```python
from build123d import *

# Parameters (mm, degrees)
SKETCH1_R           = 4
SKETCH1_R_2         = 2
BOSS_EXTRUDE1_DEPTH = 2
SKETCH3_W           = 40.799195599
SKETCH3_H           = 10.791683918
CUT_EXTRUDE1_DEPTH  = 10
SKETCH4_W           = 4.995
SKETCH4_H           = 6.450932821
BOSS_EXTRUDE2_DEPTH = 2


with BuildPart() as part:
    # Sketch1 → Boss-Extrude1 (new body)
    # profile 1 of 3: a face of its own
    with BuildSketch(Plane(origin=(0, 0, 0), x_dir=(1, 0, 0), z_dir=(0, 1, 0))):
        with BuildLine():
            ThreePointArc((26.59659241, -6.101622416), (26.022594709, -4.424555239), (26.229666852, -2.664115292))
            Line((26.229666852, -2.664115292), (10, -3.549067179))
            Line((10, -3.549067179), (-10, -3.549067179))
            Line((-10, -3.549067179), (-26.229666852, -2.664115292))
            ThreePointArc((-26.229666852, -2.664115292), (-26.057834821, -3.32225838), (-26, -4))
            ThreePointArc((-26, -4), (-26.152037529, -5.092329996), (-26.59659241, -6.101622416))
            ThreePointArc((-26.59659241, -6.101622416), (-17.96712489, -6.640913059), (-10, -10))
            Line((-10, -10), (10, -10))
            ThreePointArc((10, -10), (17.96712489, -6.640913059), (26.59659241, -6.101622416))
        make_face()
    # profile 2 of 3: a face of its own
    with BuildSketch(Plane(origin=(0, 0, 0), x_dir=(1, 0, 0), z_dir=(0, 1, 0))):
        with Locations((-30, -4)):
            Circle(SKETCH1_R)
        with Locations(Location((-30, -4, 0), (0, 0, 270))):
            Circle(SKETCH1_R_2, mode=Mode.SUBTRACT)
    # profile 3 of 3: a face of its own
    with BuildSketch(Plane(origin=(0, 0, 0), x_dir=(1, 0, 0), z_dir=(0, 1, 0))):
        with Locations((30, -4)):
            Circle(SKETCH1_R)
        with Locations(Location((30, -4, 0), (0, 0, 270))):
            Circle(SKETCH1_R_2, mode=Mode.SUBTRACT)
    extrude(amount=BOSS_EXTRUDE1_DEPTH)

    # Sketch3 → Cut-Extrude1 (cut)
    with BuildSketch(Plane(origin=(0, 2, 0), x_dir=(1, 0, 0), z_dir=(0, 1, 0))):
        with Locations((-20.3995978, -4.604158041)):
            Rectangle(SKETCH3_W, SKETCH3_H)
    extrude(amount=-CUT_EXTRUDE1_DEPTH, mode=Mode.SUBTRACT)

    # Sketch4 → Boss-Extrude2 (add)
    with BuildSketch(Plane(origin=(0, 2, 0), x_dir=(1, 0, 0), z_dir=(0, 1, 0))):
        with Locations((-2.4975, -6.774533589)):
            Rectangle(SKETCH4_W, SKETCH4_H)
    extrude(amount=-BOSS_EXTRUDE2_DEPTH)

    # Mirror3: part across plane


with BuildPart() as part_1:
    add(part.part)
    add(part.part.mirror(Plane.ZY.offset(4.995)))


solid = part_1.part
```
Verification items for the finished model (mm, model axes). A direction names the side the tool comes from. Coordinates: 2 decimals unless noted, no trailing zeros. Loops run counter-clockwise (first coordinate to the right, second up) from the corner with the lowest first, then second, coordinate; pieces in that order, holes last. Notation, with made-up numbers: (78, 37) -> (126, 37) arc R34 ccw to (126, 73) -> close; hole circle Ø11 at (12.5, 81). An arc over 180 degrees is marked (long way). Answer in a Markdown table with one row per item.
1) Access from +Z, -Z, +X, -X, +Y, -Y to the whole of each face (thin tool, end or side, straight path). Record for faces 1 (the face through (-27.84, 0.99, 6.67)), 2 (the face through (18.2, 1, 3.1)).
The answers:
| item | result |
|---|---|
| face 1 | +Z, +Y, -Y |
| face 2 | -Z, +Y, -Y |
2) Section check B-B (z = 1.25). Record the cut outline in (x, y).
The answers:
| item | result |
|---|---|
| outline | (-42.89, 0) -> (-37.09, 0) -> (-37.09, 2) -> (-42.89, 2) -> close; (27.1, 0) -> (32.9, 0) -> (32.9, 2) -> (27.1, 2) -> close |
3) Section check D-D (z = 4.25). Record the cut outline in (x, y).
The answers:
| item | result |
|---|---|
| outline | (-43.98, 0) -> (-41.97, 0) -> (-41.97, 2) -> (-43.98, 2) -> close; (-38.01, 0) -> (28.02, 0) -> (28.02, 2) -> (-38.01, 2) -> close; (31.98, 0) -> (33.99, 0) -> (33.99, 2) -> (31.98, 2) -> close |
4) Section check A-A (x = 30). Record the cut outline in (y, z), and give its area (3 significant figures).
The answers:
| item | result |
|---|---|
| outline | (0, 0) -> (2, 0) -> (2, 2) -> (0, 2) -> close; (0, 6) -> (2, 6) -> (2, 8) -> (0, 8) -> close |
| area | 8.00 mm2 |
5) Depth check by flat-ended pin: P1, Ø1, axis at y = 1, z = 2, coming from the +X side; P2, Ø1, axis at x = 22, y = 2, coming from the -Z side; P3, Ø3.5, axis at x = 30, z = 4, coming from the -Y side. Enter the tip coordinate at first touch or a pass-through.
The answers:
| item | result |
|---|---|
| P1 | stops at x = 33.71 |
| P2 | stops at z = 2.87 |
| P3 | passes through |
6) Draft check along X on faces 3 (the face through (17.85, 0.99, 6.67)), 4 (the face through (-5, 1, 10)), 5 (the face through (28, 1, 4)). Enter one of: released by +X, released by -X, zero draft, split by the parting line, or undercut.
The answers:
| item | result |
|---|---|
| face 3 | undercut |
| face 4 | zero draft |
| face 5 | undercut |
7) Section check C-C (y = 1.7). Record the cut outline in (x, z), and give its area (3 significant figures).
The answers:
| item | result |
|---|---|
| outline | (-36.59, 6.1) arc R4 ccw (long way) to (-36.22, 2.66) -> (-19.99, 3.55) -> (10, 3.55) -> (26.23, 2.66) arc R4 ccw (long way) to (26.6, 6.1) arc R25.81 cw to (10, 10) -> (-19.99, 10) arc R25.81 cw to start; hole circle Ø4 at (-39.99, 4); hole circle Ø4 at (30, 4) |
| area | 397 mm2 |
8) Scan lines: line 1 along X through (y, z) = (1.5, 4); line 2 along X through (y, z) = (0.85, 2.25); line 3 along Z through (x, y) = (-14.5, 0.2). Record each from-to range of solid material in increasing order. Write a range as from..to.
The answers:
| item | result |
|---|---|
| line 1 | x = -43.99..-41.99, -37.99..28, 32..34 |
| line 2 | x = -43.59..-40.96, -39.02..-36.39, 26.4..29.03, 30.97..33.6 |
| line 3 | z = 3.55..10 |
